Can you work these out from the drawing? Everything is in mm from the part's minimum corner. A direction names the side the tool comes from. Coordinates: 2 decimals unless noted, no trailing zeros. Order: outer loops, then holes, each group sorted by start corner. A loop starts at its lowest first (then second) coordinate and runs counter-clockwise, first axis right, second up. Notation, with made-up numbers: (-1.75, 43) - (4.25, 43) arc R18 cw to (4.25, 78) - close; hole circle Ø9 at (58, 86.5). An arc over 180 degrees is marked (long way). Answer as CSV lines item,"result". Start each with the question number.
Item 1: Imagine slicing it at D-D on x = 142.5. List the corners of the cut face in (y, z) for me, and give its area (3 significant figures).
Item 2: On a 3-axis mill with a long thin cutter (end or side, diameter ignored), from which of +Z, -Z, +X, -X, +Y, -Y can I reach the whole of each face in a straight line? I mean the marked faces 1, 2 and 3. Say none if no direction works.
Item 3: I'm going to push flat-ended pins straight in: pin 1 (10 mm diameter, centred on x = 113.5, z = 23, fed in from -Y); pin 2 (3 mm diameter, centred on y = 57.5, z = 21.5, fed in from +X); pin 3 (2 mm diameter, centred on x = 92, y = 50, fed in from -Z). Where does each tip first touch, or does it pass through?
Item 4: Imagine slicing it at C-C on x = 32.5. List the corners of the cut face in (y, z) for me, and give its area (3 significant figures).
Item 5: Imagine slicing it at A-A on z = 40. List the corners of the cut face in (x, y) for me, and give its area (3 significant figures).
Item 6: I need wall thicknesses on line 1 (X direction, y = 9, z = 41); line 2 (X direction, y = 31.5, z = 62.5); line 3 (Y direction, x = 117, z = 39). Which ranges of each line are inside material? Lowest first, please.
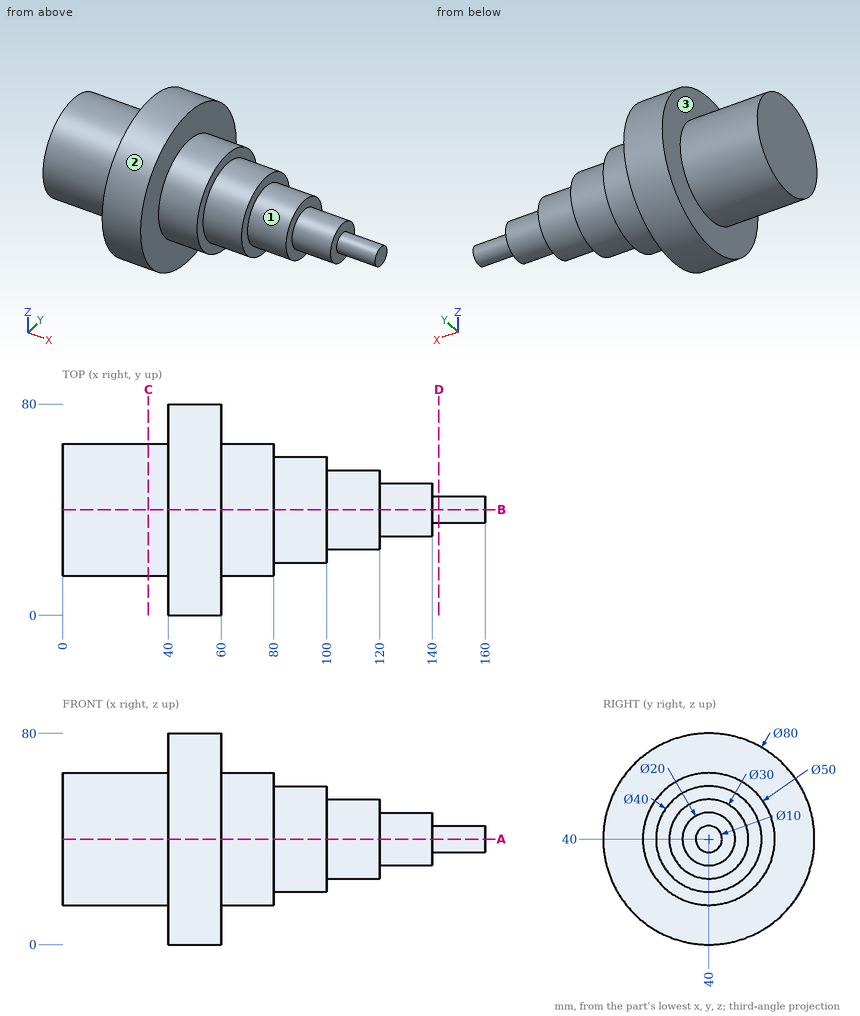
Responses:
1,outline,"circle Ø10 at (40, 40)"
1,area,"78.5 mm^2"
2,face 1,"+X"
2,face 2,"+X, -X"
2,face 3,"-X"
3,pin 1,"stops at y = 31"
3,pin 2,"stops at x = 80"
3,pin 3,"stops at z = 22.14"
4,outline,"circle Ø50 at (40, 40)"
4,area,"1,960 mm^2"
5,outline,"(0, 15) - (40, 15) - (40, 0) - (60, 0) - (60, 15) - (80, 15) - (80, 20) - (100, 20) - (100, 25) - (120, 25) - (120, 30) - (140, 30) - (140, 35) - (160, 35) - (160, 45) - (140, 45) - (140, 50) - (120, 50) - (120, 55) - (100, 55) - (100, 60) - (80, 60) - (80, 65) - (60, 65) - (60, 80) - (40, 80) - (40, 65) - (0, 65) - close"
5,area,"6,600 mm^2"
6,line 1,"x = 40 to 60"
6,line 2,"x = 0 to 80"
6,line 3,"y = 25.03 to 54.97"
